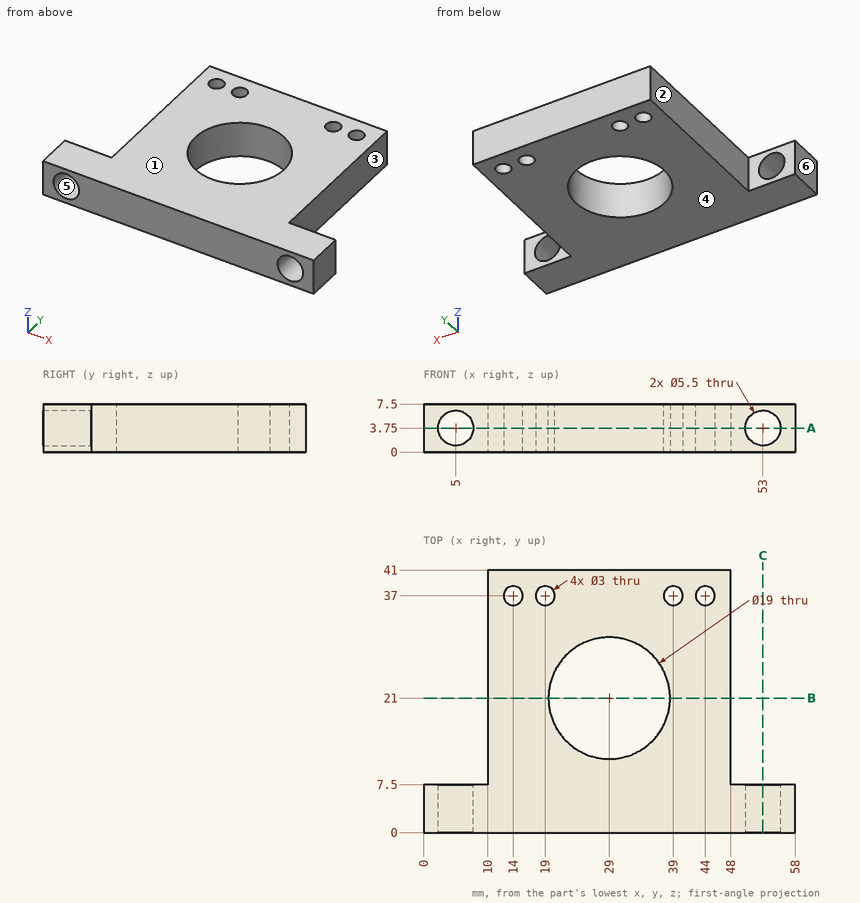
Check sheet for the drawn part. Datum: minimum x, y, z corner. Units: mm. A direction names the side the tool comes from. Round coordinates to 2 decimals unless told otherwise and drop trailing zeros. Order: outer loops, then holes, each group sorted by start corner. A loop starts at its lowest first (then second) coordinate and runs counter-clockwise, first axis right, second up.
1) Section check A-A (z = 3.75). Record the boundary of the cut face in (x, y).
2) Go/stop test with flat-tipped pins: pin 1 Ø3 at (y, z) = (14, 6) entering from -X; pin 2 Ø1 at (y, z) = (12.5, 1.5) entering from +X. Record where each tip stops, or that it passes through.
3) Tool access check on the marked faces 1, 2 and 3. Record the directions out of +Z, -Z, +X, -X, +Y, -Y that give a thin tool (end or side, any length) a straight path to the whole face; none if there is none.
4) Scan lines: line 1 (Z direction, x = 53, y = 2.75); line 2 (Y direction, x = 39, z = 5.25); line 3 (X direction, y = 3, z = 4). Record each from-to range of solid material in increasing order.
5) Mould release check, pull along X, two halves, no side actions. Record for the marked faces 4, 5 and 6: +X half, -X half, draft (parallel to the pull), parting line (faces both ways), or undercut.
6) Section check C-C (x = 53). Record the boundary of the cut face in (y, z), and give its area (3 significant figures).
7) Section check B-B (y = 21). Record the boundary of the cut face in (x, z), and give its area (4 significant figures).
Result:
1. outline: (0, 0) - (2.25, 0) - (2.25, 7.5) - (0, 7.5) - close; (7.75, 0) - (50.25, 0) - (50.25, 7.5) - (48, 7.5) - (48, 41) - (10, 41) - (10, 7.5) - (7.75, 7.5) - close; (55.75, 0) - (58, 0) - (58, 7.5) - (55.75, 7.5) - close; hole circle Ø3 at (14, 37); hole circle Ø3 at (19, 37); hole circle Ø19 at (29, 21); hole circle Ø3 at (39, 37); hole circle Ø3 at (44, 37)
2. pin 1: stops at x = 10
2. pin 2: stops at x = 48
3. face 1: +Z, +X, -X, +Y, -Y
3. face 2: +Z, -Z, -X, +Y
3. face 3: +Z, -Z, +X, +Y
4. line 1: z = 0 to 1, 6.5 to 7.5
4. line 2: y = 0 to 35.5, 38.5 to 41
4. line 3: x = 0 to 2.26, 7.74 to 50.26, 55.74 to 58
5. face 4: draft
5. face 5: undercut
5. face 6: -X half
6. outline: (0, 0) - (7.5, 0) - (7.5, 1) - (0, 1) - close; (0, 6.5) - (7.5, 6.5) - (7.5, 7.5) - (0, 7.5) - close
6. area: 15.0 mm2
7. outline: (10, 0) - (19.5, 0) - (19.5, 7.5) - (10, 7.5) - close; (38.5, 0) - (48, 0) - (48, 7.5) - (38.5, 7.5) - close
7. area: 142.5 mm2
